Autodesk Inventor part; units mm, degrees
ref_plane "YZ Plane" through (0, 0, 0) normal (1, 0, 0) x (0, 1, 0)
ref_plane "XZ Plane" through (0, 0, 0) normal (0, 1, 0) x (-1, 0, 0)
ref_plane "XY Plane" through (0, 0, 0) normal (0, 0, 1) x (1, 0, 0)
sketch "Sketch1" plane through (0, 0, 0) normal (0, 0, 1) x (1, 0, 0)
  line L0 (0, 0) -> (27.815, 0)
  line L1 (27.815, 0) -> (27.815, 338.525)
  line L2 (27.815, 338.525) -> (0, 338.525)
  line L3 (0, 338.525) -> (0, 0)
  dimension "d0" = 27.815
  dimension "d1" = 338.525
extrude "Plate1" add sketch "Sketch1" along normal blind 0.5
sketch "Sketch2" plane through (28.8794, 338.525, 3.057) normal (0.7095707, 0, 0.7046342) x (0, 1, 0)
  line L0 (-338.525, 0) -> (0, 0)
  line L1 (0, 0) -> (0, 27.8153)
  line L2 (0, 27.8153) -> (-338.525, 27.8153)
  line L3 (-338.525, 27.8153) -> (-338.525, 0)
edge flange "Flange1" height 32.62 angle 134.8 thickness 0.5 bend radius 1.5 thickness toward (0.7095707, 0, 0.7046342) relief tear relief width 0.5 relief depth 0.25 edges at (27.815, 169.2625, 0.5) wall of the first edge with corners at (28.8794, 0, 3.057) (28.8794, 338.525, 3.057) (9.2797, 338.525, 22.7939) (9.2797, 0, 22.7939)
bend "Bend1"
corner "Corner1"
sketch "Sketch3" plane through (9.6345, 0, 23.1462) normal (0.7095707, 0, 0.7046342) x (0.7046342, 0, -0.7095707)
  line L0 (0, 338.525) -> (27.8153, 338.525)
  line L1 (27.8153, 0) -> (0, 0)
  line L2 (0, 0) -> (3, 0) construction
  line L3 (3, 0) -> (3, 3.175) construction
  line L4 (0, 338.525) -> (3, 338.525)
  line L5 (3, 338.525) -> (3, 335.35) construction
  circle A0 centre (3, 335.35) radius 1.25
  line L6 (3, 3.175) -> (3, 3.35) construction
  circle A1 centre (3, 3.35) radius 1.25
  point P0 (9.635, 0)
  dimension "d13" = 3
  dimension "d14" = 3.175
  dimension "d16" = 3
  dimension "d17" = 3.175
  dimension "d18" = 2.5
  dimension "d34" = 0.175
  dimension "d35" = 2.5
extrude "Extrusion1" cut sketch "Sketch3" against normal blind 10
sketch "Sketch4" plane through (0, 0, 0) normal (0, 0, -1) x (-1, 0, 0)
  line L0 (0, 0) -> (-27.815, 0)
  line L1 (0, 0) -> (-3, 0) construction
  line L2 (-3, 0) -> (-3, 3.175) construction
  line L3 (0, 338.525) -> (-3, 338.525) construction
  line L4 (0, 338.525) -> (-27.815, 338.525) construction
  line L5 (-3, 338.525) -> (-3, 335.35) construction
  circle A0 centre (-3, 335.35) radius 1.25
  line L6 (-3, 3.175) -> (-3, 3.35) construction
  circle A1 centre (-3, 3.35) radius 1.25
  dimension "d21" = 3
  dimension "d22" = 3.175
  dimension "d24" = 3
  dimension "d25" = 3.175
  dimension "d26" = 2.5
  dimension "d32" = 0.175
  dimension "d33" = 2.5
extrude "Extrusion2" cut sketch "Sketch4" against normal blind 10
sketch "Sketch5" plane through (0, 0, 0) normal (0, 0, -1) x (-1, 0, 0)
  line L0 (0, 0) -> (-49.0059, 0)
  line L1 (-49.0059, 0) -> (-49.0059, 0.175)
  line L2 (-49.0059, 0.175) -> (0, 0.175)
  line L3 (0, 0.175) -> (0, 0)
  dimension "d29" = 0.175
extrude "Extrusion3" cut sketch "Sketch5" against normal blind 100
sketch "Sketch6" plane through (0, 338.525, 0) normal (0, 1, 0) x (1, 0, 0)
  line L0 (0, -0.5) -> (27.815, -0.5)
  line L1 (27.815, 0) -> (27.815, -0.5)
  line L2 (27.815, 0) -> (0, 0)
  line L3 (0, 0) -> (0, -0.5)
extrude "Extrusion4" add sketch "Sketch6" along normal blind 30.87
sketch "Sketch7" plane through (27.815, 338.525, 0.5) normal (0, 1, 0) x (1, 0, 0)
  line L0 (1.4191, -2.9093) -> (1.0644, -2.557)
  arc A0 (1.4191, -2.9093) -> (0, 0.5) centre (0, -1.5) ccw
  line L1 (0, 0.5) -> (0, 0)
  arc A1 (1.0644, -2.557) -> (0, 0) centre (0, -1.5) ccw
  point P0 (-27.815, 0.5)
extrude "Extrusion5" add sketch "Sketch7" along normal blind 30.87
sketch "Sketch8" plane through (9.2797, 338.525, 22.7939) normal (0, 1, 0) x (0.7095707, 0, 0.7046342)
  line L0 (0.5, 27.8153) -> (0, 27.8153)
  line L1 (0, 0) -> (0, 27.8153)
  line L2 (0, 0) -> (0.5, 0)
  line L3 (0.5, 0) -> (0.5, 27.8153)
  point P0 (-22.646, 9.635)
extrude "Extrusion6" add sketch "Sketch8" along normal blind 30.87
sketch "Sketch9" plane through (29.2341, 0.175, 3.4093) normal (0.7095707, 0, 0.7046342) x (0.7046342, 0, -0.7095707)
  circle A0 centre (-24.8153, 335.175) radius 1.25
  point P0 (-18.1803, -0.175)
extrude "Extrusion7" add sketch "Sketch9" against normal up to surface (0.5 mm away)
sketch "Sketch10" plane through (0, 0, 0) normal (0, 0, -1) x (-1, 0, 0)
  circle A0 centre (-3, 335.35) radius 1.25
  point P0 (0, 0)
extrude "Extrusion8" add sketch "Sketch10" against normal up to surface (0.5 mm away)
sketch "Sketch11" plane through (0, 0, 0) normal (0, 0, -1) x (-1, 0, 0)
  line L0 (0, 0.175) -> (0, 369.395)
  line L1 (0, 369.395) -> (0, 366.22) construction
  line L2 (0, 366.22) -> (-3, 366.22) construction
  circle A0 centre (-3, 366.22) radius 1.5
  point P0 (0, 0)
  dimension "d46" = 3.175
  dimension "d47" = 3
  dimension "d48" = 3
extrude "Extrusion9" cut sketch "Sketch11" against normal blind 30.87
sketch "Sketch12" plane through (29.2341, 0.175, 3.4093) normal (0.7095707, 0, 0.7046342) x (0.7046342, 0, -0.7095707)
  line L0 (-27.8153, 0) -> (-27.8153, 369.22)
  line L1 (-27.8153, 369.22) -> (-27.8153, 366.045) construction
  line L2 (-27.8153, 0) -> (-27.8153, 369.22) construction
  line L3 (-27.8153, 366.045) -> (-24.8153, 366.045) construction
  circle A0 centre (-24.8153, 366.045) radius 1.5
  point P0 (-18.1803, -0.175)
  dimension "d51" = 3.175
  dimension "d52" = 3
  dimension "d53" = 3
extrude "Extrusion10" cut sketch "Sketch12" against normal blind 30.87
equation "\"d2\" = Thickness"
equation "\"d3\" = BendReliefWidth"
equation "\"d4\" = BendReliefDepth"
equation "\"d5\" = MinimumRemnant"
equation "\"d6\" = TransitionRadius"
equation "\"d10\" = CornerReliefSize"
equation "\"d11\" = GapSize"
equation "\"d12\" = JacobiRadiusSize"
equation "\"BendRadius\" = Thickness"
equation "\"BendReliefWidth\" = Thickness"
equation "\"BendReliefDepth\" = 0.5 * Thickness"
equation "\"CornerReliefSize\" = 4 * Thickness"
equation "\"MinimumRemnant\" = 2 * Thickness"
equation "\"TransitionRadius\" = BendRadius"
equation "\"JacobiRadiusSize\" = BendRadius"
equation "\"GapSize\" = Thickness"
properties part number "sideplate part 3" material "Aluminum 6061"
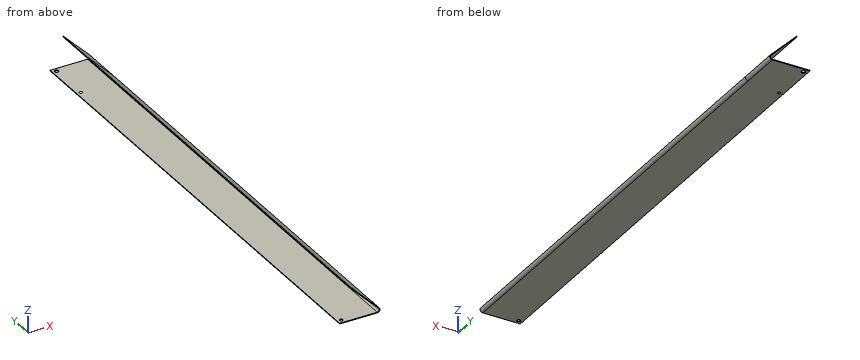
Design review of the part built by this model. Coordinates are the model's own, in mm. Coordinates: 2 decimals unless noted, no trailing zeros. Write each loop counter-clockwise with the first axis right and the second up, starting at its lowest first coordinate (ties: lowest second). Pieces come first, ordered by that corner, then holes. Notation, with made-up numbers: (12.5, 55) -> (26.5, 55) arc R25 cw to (26.5, 85) -> close; hole circle Ø10 at (87, 49). An arc over 180 degrees is marked (long way). Write each question's results on one line, items separated by ' | '. Start each with the question number.
(1) Take a section at A-A on y = 260. Write out the cut boundary in (x, z) (3 decimals), and give its area (3 significant figures).
(2) Take a section at B-B on x = 17.75. Write out the cut boundary in (y, z) (3 decimals).
(3) For line 1 along Y through (x, z) = (3, 0.25) (3 decimals); line 2 along X through (y, z) = (55, 2); line 3 along X through (y, z) = (366.22, 0.3), list the stretches that pass through material, from the lowest coordinate up. Write a range as from..to.
(4) Clearance check with flat-ended pins moving along their axes: P1, Ø1.5, axis at x = 3, y = 3.35, coming from the +Z side; P2, Ø2, axis at y = 144.5, z = 16.5, coming from the +X side; P3, Ø1.5, axis at y = 305.5, z = 4.5, coming from the +X side; P4, Ø3, axis at x = 11.5, y = 284.5, coming from the +Z side. State where each tip first meets the part, or that it passes through.
(5) Take a section at C-C on z = 13.75. Write out the cut boundary in (x, y) (3 decimals).
Results found:
1) outline: (0, 0) -> (27.815, 0) arc R2 ccw to (29.234, 3.409) -> (9.634, 23.146) -> (9.28, 22.794) -> (28.879, 3.057) arc R1.5 cw to (27.815, 0.5) -> (0, 0.5) -> close | area: 29.9 mm2
2) outline: (0.175, 0) -> (369.395, 0) -> (369.395, 0.5) -> (0.175, 0.5) -> close; (0.175, 14.264) -> (369.395, 14.264) -> (369.395, 14.974) -> (0.175, 14.974) -> close
3) line 1: y = 0.175..2.1, 4.6..364.72, 367.72..369.395 | line 2: x = 29.32..29.82 | line 3: x = 0..1.5, 4.5..28.87
4) P1: passes through | P2: stops at x = 17.23 | P3: stops at x = 28.9 | P4: stops at z = 22.78
5) outline: (18.261, 0.175) -> (18.965, 0.175) -> (18.965, 369.395) -> (18.261, 369.395) -> close
